CAD build for the part. Positions are in the model's coordinates, mm. A direction names the side the tool comes from. Coordinates: 2 decimals unless noted, no trailing zeros. Loops run counter-clockwise (first coordinate to the right, second up) from the corner with the lowest first, then second, coordinate; pieces in that order, holes last.
1) Saw through at B-B, the plane z = 0.7. Write the cut outline in (x, y).
2) Saw through at D-D, the plane y = 35. Write the cut outline in (x, z), and give its area (3 significant figures).
3) Two-plate mould, pull along Y, no slides. Class faces 4 (the cylindrical face through (55.451, 23.426, 0.438)), 5 (the cylindrical face through (52.76, 24.98, 0.44)), 6 (the cylindrical face through (53.53, 55.26, 0.44)), 7 (the cylindrical face through (55.169, 15.102, 0.438)): +Y half, -Y half, draft (parallel to the pull), parting line (faces both ways), or undercut.
4) Saw through at C-C, the plane x = 59.5. Write the cut outline in (y, z).
5) Saw through at A-A, the plane y = 40.5. Write the cut outline in (x, z), and give its area (3 significant figures).
6) Which spindle directions (+Z, -Z, +X, -X, +Y, -Y) get a long thin tool onto all of the face, cutting with end or side? Do faces 1 (the flat face through (55.717, 32.816, 0.438)), 2 (the flat face through (58.607, 18.8, 0.4)), 3 (the flat face through (56, 32, 0)). Say none if no direction does.
7) Wall check: line 1 along Y through (x, z) = (56.75, 0.25); line 2 along X through (y, z) = (19, 0.6); line 3 along X through (y, z) = (48.5, 0.25). Give the ranges that are in metal, low to high.
```python
from build123d import *

# Parameters (mm, degrees)
SKETCH1_R           = 1.27
BOSS_EXTRUDE3_DEPTH = 0.889
SKETCH3_R           = 2.032
CUT_EXTRUDE1_DEPTH  = 1.889
CUT_EXTRUDE2_DEPTH  = 12.7


with BuildPart() as part:
    # Sketch1 → Boss-Extrude3 (new body)
    with BuildSketch(Plane.XY):
        with BuildLine():
            Line((54.54799083, 56.616289575), (56.611609417, 46.195015712))
            ThreePointArc((56.611609417, 46.195015712), (56.978037984, 44.693364942), (58.298969551, 43.890641624))
            Line((58.298969551, 43.890641624), (60.203091121, 20.328922191))
            Line((60.203091121, 20.328922191), (58.607476528, 20.19997387))
            Line((58.607476528, 20.19997387), (58.607476528, 17.442451046))
            ThreePointArc((58.607476528, 17.442451046), (55.106284247, 15.101864773), (51.605091967, 17.442451046))
            Line((51.605091967, 17.442451046), (51.481381748, 24.727035664))
            ThreePointArc((51.481381748, 24.727035664), (52.781095987, 24.992110323), (53.724469669, 25.924616503))
            ThreePointArc((53.724469669, 25.924616503), (55.527536206, 26.293339608), (56.052311948, 28.057316955))
            Line((56.052311948, 28.057316955), (55.371384499, 37.710464906))
            Line((55.371384499, 37.710464906), (53.003003997, 39.540899235))
            ThreePointArc((53.003003997, 39.540899235), (52.354767278, 46.624659681), (52.993412204, 53.709291327))
            ThreePointArc((52.993412204, 53.709291327), (53.543144587, 55.284481319), (54.54799083, 56.616289575))
        make_face()
        with Locations((55.596905374, 41.346801264)):
            Circle(SKETCH1_R, mode=Mode.SUBTRACT)
        with Locations((54.27760068, 23.912500713)):
            Circle(SKETCH1_R, mode=Mode.SUBTRACT)
    extrude(amount=BOSS_EXTRUDE3_DEPTH)

    # Sketch3 → Cut-Extrude1 (cut, through all)
    with BuildSketch(Plane.XY.offset(0.889)):
        with Locations((55.106284247, 18.890806819)):
            Circle(SKETCH3_R)
    extrude(amount=-CUT_EXTRUDE1_DEPTH, mode=Mode.SUBTRACT)

    # Sketch4 → Cut-Extrude2 (cut)
    with BuildSketch(Plane(origin=(-8.897590356, 44.932831299, 0), x_dir=(0.980952451, 0.19424801, 0), z_dir=(-0.19424801, 0.980952451, 0))):
        Polygon((64.506586873, 0), (64.506586873, -0.889), (63.993322484, -0.889), align=None)
    extrude(amount=-CUT_EXTRUDE2_DEPTH, mode=Mode.SUBTRACT)


solid = part.part
```
Data:
1. outline: (51.48, 24.73) - (51.61, 17.44) arc R3.79 ccw to (58.61, 17.44) - (58.61, 20.2) - (60.2, 20.33) - (58.3, 43.89) arc R2.02 cw to (56.8, 44.99) - (56.45, 44.93) - (54.21, 56.25) arc R5.39 ccw to (52.99, 53.71) arc R39.32 ccw to (53, 39.54) - (55.37, 37.71) - (56.05, 28.06) arc R1.79 cw to (53.72, 25.92) arc R2.33 cw to start; hole circle Ø2.54 at (54.28, 23.91); hole circle Ø4.06 at (55.11, 18.89); hole circle Ø2.54 at (55.6, 41.35)
2. outline: (55.56, 0) - (59.02, 0) - (59.02, 0.89) - (55.56, 0.89) - close
2. area: 3.07 mm2
3. face 4: undercut
3. face 5: undercut
3. face 6: +Y half
3. face 7: -Y half
4. outline: (20.27, 0) - (29.03, 0) - (29.03, 0.89) - (20.27, 0.89) - close
5. outline: (52.84, 0) - (54.65, 0) - (54.65, 0.89) - (52.84, 0.89) - close; (56.54, 0) - (58.57, 0) - (58.57, 0.89) - (56.54, 0.89) - close
5. area: 3.41 mm2
6. face 1: +Z, -Z, -X
6. face 2: +Z, -Z, +X, -Y
6. face 3: -Z, +X, -X, +Y, -Y
7. line 1: y = 15.48 to 17.7, 20.09 to 40.81, 41.88 to 44.99
7. line 2: x = 51.58 to 53.08, 57.14 to 58.61
7. line 3: x = 52.4 to 56.01
